from build123d import *

# Parameters (mm, degrees)
F2_DEPTH = 25.4
F3_DEPTH = 25.4


with BuildPart() as f2:
    # F0 (on Front) → F2 (new body)
    with BuildSketch(Plane.XZ):
        with BuildLine():
            ThreePointArc((36.588859, -19.241439), (26.227151, -0.024717), (36.62506, 19.172441))
            ThreePointArc((36.62506, 19.172441), (9.628766, 40.202791), (-23.965633, 33.68421))
            ThreePointArc((-23.965633, 33.68421), (-27.205101, -31.126516), (36.588859, -19.241439))
        make_face()
    extrude(amount=F2_DEPTH)

    # F0 (on Front) → F3 (join)
    with BuildSketch(Plane.XZ):
        with BuildLine():
            ThreePointArc((36.588859, -19.241439), (40.13448, -9.909645), (41.339782, 0))
            ThreePointArc((41.339782, 0), (40.143801, 9.871817), (36.62506, 19.172441))
            ThreePointArc((36.62506, 19.172441), (26.227151, -0.024717), (36.588859, -19.241439))
        make_face()
        with BuildLine():
            ThreePointArc((36.588859, -19.241439), (26.227151, -0.024717), (36.62506, 19.172441))
            ThreePointArc((36.62506, 19.172441), (9.628766, 40.202791), (-23.965633, 33.68421))
            ThreePointArc((-23.965633, 33.68421), (-27.205101, -31.126516), (36.588859, -19.241439))
        make_face()
        with BuildLine():
            ThreePointArc((-23.965633, 33.68421), (9.628766, 40.202791), (36.62506, 19.172441))
            Line((36.62506, 19.172441), (36.62506, 76.793261))
            Line((36.62506, 76.793261), (-23.965633, 33.68421))
        make_face()
    extrude(amount=F3_DEPTH)


solid = f2.part
CAD build for the part. Positions are in the model's coordinates, mm. A direction names the side the tool comes from. Round coordinates to 2 decimals unless told otherwise and drop trailing zeros. Order: outer loops, then holes, each group sorted by start corner. A loop starts at its lowest first (then second) coordinate and runs counter-clockwise, first axis right, second up. Notation, with made-up numbers: (84, 78.5) -> (102, 78.5) arc R10 ccw to (102, 82.5) -> close; hole circle Ø5 at (53.25, -15). An arc over 180 degrees is marked (long way). Write each question's results on one line, items separated by ' | '.
1. Flat gauge pins, fed straight in: P1, Ø1.5, axis at x = 0.5, y = -15.5, coming from the +Z side; P2, Ø2, axis at y = -12, z = -16, coming from the +X side; P3, Ø6, axis at x = -19, y = -9.5, coming from the -Z side. Where does each tip first touch, or does it go through?
Findings below:
P1: stops at z = 51.62 | P2: stops at x = 38.52 | P3: stops at z = -38.12
2. 3-axis set-ups, long thin cutter, end or side, ignore diameter. For faces 1 (the face through (6.75, -12.52, 55.54)), 2 (the face through (36.625, -13, 48)): which of +Z, -Z, +X, -X, +Y, -Y reach the whole face in a straight line?
Findings below:
face 1: +Z, -X, +Y, -Y | face 2: +Z, +X, +Y, -Y
3. Cut at A-A (y = -16). Give the cut face in (x, z), plus the area to 3 significant figures.
Findings below:
outline: (-23.97, 33.68) arc R41.34 ccw (long way) to (36.59, -19.24) arc R41.34 ccw to (41.34, 0) arc R41.34 ccw to (36.63, 19.17) -> (36.63, 76.79) -> close | area: 6,500 mm²
4. Cut at B-B (z = 68). Give the cut face in (x, y), plus the area to 3 significant figures.
Findings below:
outline: (24.27, -25.4) -> (36.63, -25.4) -> (36.63, 0) -> (24.27, 0) -> close | area: 314 mm²
5. Cut at C-C (x = 0). Give the cut face in (y, z), plus the area to 3 significant figures.
Findings below:
outline: (-25.4, -41.34) -> (0, -41.34) -> (0, 50.74) -> (-25.4, 50.74) -> close | area: 2,340 mm²
6. Wall check: line 1 along X through (y, z) = (-10.75, 71.5); line 2 along X through (y, z) = (-20.5, 7); line 3 along Z through (x, y) = (-34, -7). Give the ranges that are in metal, low to high. Write a range as [from, to].
Findings below:
line 1: x = [29.19, 36.63] | line 2: x = [-40.74, 40.74] | line 3: z = [-23.52, 23.52]
